Input: part model. Units: mm. Frame: model coordinates. Give positions to 0.01 mm unless a question says otherwise; leave off trailing zeros. Loops run counter-clockwise (first coordinate to the right, second up) from the corner with the lowest first, then second, coordinate; pieces in that order, holes last. Notation, with made-up numbers: (4, -5) - (38, -5) arc R24 cw to (38, 28) - close; hole circle Ø4 at (82.5, 42). An arc over 180 degrees is marked (long way). Answer as a JSON object with one key per item and string values. Group by question number.
(1) Material intervals for L1, parallel to X at y = 5.25, z = -20.5; L2, parallel to Z at x = 36.5, y = 4; L3, parallel to X at y = 14, z = 3, sorted ascending.
(2) Section query B-B (z = -12.5). Return loops of the section in (x, y).
(3) Pin query (flat end, axial travel): P1, Ø4, axis at y = 22, z = -21, coming from the -X side. Return the tip coordinate at first contact, or that it passes through.
(4) Section query A-A (y = 27.5). Return loops of the section in (x, z), plus the area to 3 significant figures.
```python
from build123d import *

# Parameters (mm, degrees)
SKETCH1_W                      = 104.5
SKETCH1_H                      = 59.5
BOSS_EXTRUDE1_DEPTH            = 30.25
SKETCH2_R                      = 2
BOSS_EXTRUDE2_DEPTH            = 10
M4_CLEARANCE_HOLE1_D           = 4.5
M4_CLEARANCE_HOLE1_DEPTH       = 10
M4_CLEARANCE_HOLE1_CSINK_D     = 4.55
M4_CLEARANCE_HOLE1_CSINK_ANGLE = 90
M4_CLEARANCE_HOLE1_TIP         = 1.351936393


with BuildPart() as part:
    # Sketch1 → Boss-Extrude1 (new body)
    with BuildSketch(Plane(origin=(0, 0, 0), x_dir=(1, 0, 0), z_dir=(0, 1, 0))):
        Rectangle(SKETCH1_W, SKETCH1_H)
    extrude(amount=BOSS_EXTRUDE1_DEPTH)

    # Sketch2 → Boss-Extrude2 (add)
    with BuildSketch(Plane.ZY.offset(52.25)):
        with Locations(Location((0, 11.6, 0), (0, 0, 180))):
            Circle(SKETCH2_R)
    extrude(amount=BOSS_EXTRUDE2_DEPTH)

    # M4 Clearance Hole1
    with Locations(Plane(origin=(0, 0, 0), x_dir=(-1, 0, 0), z_dir=(0, -1, 0))):
        with Locations((36.5, 20.5), (-36.5, 20.5), (-36.5, -20.5), (36.5, -20.5)):
            CounterSinkHole(M4_CLEARANCE_HOLE1_D / 2, M4_CLEARANCE_HOLE1_CSINK_D / 2, depth=M4_CLEARANCE_HOLE1_DEPTH, counter_sink_angle=M4_CLEARANCE_HOLE1_CSINK_ANGLE)
            with Locations((0, 0, -(M4_CLEARANCE_HOLE1_DEPTH + M4_CLEARANCE_HOLE1_TIP / 2))):  # 118° drill point
                Cone(0, M4_CLEARANCE_HOLE1_D / 2, M4_CLEARANCE_HOLE1_TIP, mode=Mode.SUBTRACT)


solid = part.part
```
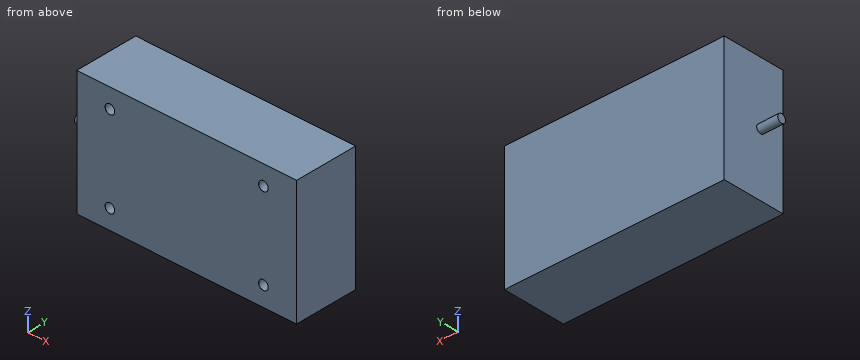
Recorded:
{
 "1": {"L1": "x = -52.25 to -38.75, -34.25 to 34.25, 38.75 to 52.25", "L2": "z = -29.75 to -22.75, -18.25 to 18.25, 22.75 to 29.75", "L3": "x = -52.25 to 52.25"},
 "2": {"outline": "(-52.25, 0) - (52.25, 0) - (52.25, 30.25) - (-52.25, 30.25) - close"},
 "3": {"P1": "stops at x = -52.25"},
 "4": {"outline": "(-52.25, -29.75) - (52.25, -29.75) - (52.25, 29.75) - (-52.25, 29.75) - close", "area": "6,220 mm^2"}
}
